Print and shaded views of the part. All mm, measured from the part's lowest x, y and z. A direction names the side the tool comes from. Round coordinates to 2 decimals unless told otherwise and drop trailing zeros. Order: outer loops, then holes, each group sorted by start corner. A loop starts at its lowest first (then second) coordinate and runs counter-clockwise, first axis right, second up. Notation, with made-up numbers: (9.25, 21.25) - (63.25, 21.25) arc R20 ccw to (63.25, 55.25) - close; hole circle Ø3 at (-7.5, 24). An arc over 180 degrees is marked (long way). Write item = value, one per line.
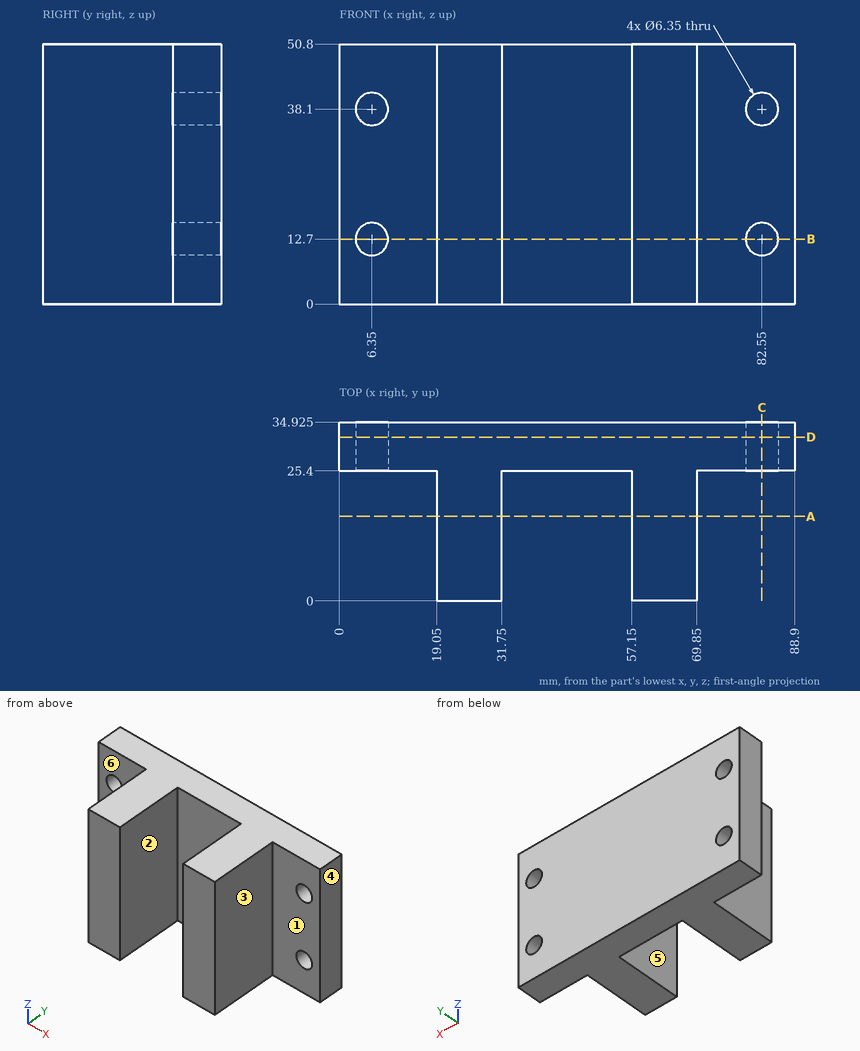
(1) Band-saw the part on B-B on z = 12.7. List the corners of the cut face in (x, y) (3 decimals).
Solved:
outline = (0, 25.4) - (3.175, 25.4) - (3.175, 34.925) - (0, 34.925) - close; (9.525, 25.4) - (19.05, 25.4) - (19.05, 0) - (31.75, 0) - (31.75, 25.4) - (57.15, 25.4) - (57.15, 0) - (69.85, 0) - (69.85, 25.4) - (79.375, 25.4) - (79.375, 34.925) - (9.525, 34.925) - close; (85.725, 25.4) - (88.9, 25.4) - (88.9, 34.925) - (85.725, 34.925) - close
(2) Probe line 1 along Z through (x, y) = (82.55, 32.25) (3 decimals); line 2 along X through (y, z) = (32.5, 38.1) (3 decimals); line 3 along X through (y, z) = (10, 9). List the from-to ranges inside material, lowest first.
Solved:
line_1 = 0 to 9.525, 15.875 to 34.925, 41.275 to 50.8
line_2 = 0 to 3.175, 9.525 to 79.375, 85.725 to 88.9
line_3 = 19.05 to 31.75, 57.15 to 69.85
(3) Band-saw the part on C-C on x = 82.55. List the corners of the cut face in (y, z) (3 decimals).
Solved:
outline = (25.4, 0) - (34.925, 0) - (34.925, 9.525) - (25.4, 9.525) - close; (25.4, 15.875) - (34.925, 15.875) - (34.925, 34.925) - (25.4, 34.925) - close; (25.4, 41.275) - (34.925, 41.275) - (34.925, 50.8) - (25.4, 50.8) - close
(4) Drop flat-ended pins along their axis: pin 1 (7.5 mm diameter, centred on y = 13, z = 32, fed in from +X); pin 2 (5 mm diameter, centred on y = 16.5, z = 12.5, fed in from -X); pin 3 (5.5 mm diameter, centred on x = 10, z = 30.5, fed in from -Y); pin 4 (4 mm diameter, centred on x = 6.35, z = 38.1, fed in from +Y). Give the stop position or say it passes through.
Solved:
pin_1 = 69.85
pin_2 = 19.05
pin_3 = 25.4
pin_4 = through
(5) Band-saw the part on D-D on y = 32. List the corners of the cut face in (x, z) (3 decimals), plus the area to 3 significant figures.
Solved:
outline = (0, 0) - (88.9, 0) - (88.9, 50.8) - (0, 50.8) - close; hole circle Ø6.35 at (6.35, 12.7); hole circle Ø6.35 at (6.35, 38.1); hole circle Ø6.35 at (82.55, 12.7); hole circle Ø6.35 at (82.55, 38.1)
area = 4,390 mm²
(6) Pull direction X, two halves, no side cores. Call the marked faces 1, 2 and 3: released by +X, released by -X, zero draft, split by the parting line, or undercut.
Solved:
face_1 = zero draft
face_2 = undercut
face_3 = released by +X
(7) Band-saw the part on A-A on y = 16.5. List the corners of the cut face in (x, z).
Solved:
outline = (19.05, 0) - (31.75, 0) - (31.75, 50.8) - (19.05, 50.8) - close; (57.15, 0) - (69.85, 0) - (69.85, 50.8) - (57.15, 50.8) - close
(8) Tool access for the marked faces 4, 5 and 6: list every direction of +Z, -Z, +X, -X, +Y, -Y with a clear straight run to the whole face (end or side of a thin tool).
Solved:
face_4 = +Z, -Z, +X, +Y, -Y
face_5 = +Z, -Z, -Y
face_6 = +Z, -Z, -X, -Y
